Verification items for the finished model (mm, model axes). Give positions to 0.01 mm unless a question says otherwise; leave off trailing zeros. Write each loop counter-clockwise with the first axis right and the second up, starting at its lowest first coordinate (ties: lowest second). Pieces come first, ordered by that corner, then holes. Notation, with made-up numbers: (24, 82) - (77, 82) arc R22 cw to (77, 113) - close; hole circle Ø3 at (-22, 51). An arc over 180 degrees is marked (long way). Put each result on its own line as item: value.
from build123d import *

# Parameters (mm, degrees)
SKETCH_R        = 17.5
SKETCH_R_2      = 8.85
SKETCH_R_3      = 2.6
PAD_DEPTH       = 5.2
SKETCH001_R     = 17.5
SKETCH001_R_2   = 8.85
PAD001_DEPTH    = 0.2
CHAMFER_SIZE    = 0.25
CHAMFER001_SIZE = 0.25


with BuildPart() as part:
    # Sketch → Pad (new body)
    with BuildSketch(Plane.XY):
        Circle(SKETCH_R)
        Circle(SKETCH_R_2, mode=Mode.SUBTRACT)
        with Locations((12.5, 0)):
            Circle(SKETCH_R_3, mode=Mode.SUBTRACT)
        with Locations((-12.5, 0)):
            Circle(SKETCH_R_3, mode=Mode.SUBTRACT)
        with Locations((-6.25, 10.825318)):
            Circle(SKETCH_R_3, mode=Mode.SUBTRACT)
        with Locations((6.25, 10.825318)):
            Circle(SKETCH_R_3, mode=Mode.SUBTRACT)
        with Locations((-6.25, -10.825318)):
            Circle(SKETCH_R_3, mode=Mode.SUBTRACT)
        with Locations((6.25, -10.825318)):
            Circle(SKETCH_R_3, mode=Mode.SUBTRACT)
    extrude(amount=PAD_DEPTH)

    # Sketch001 → Pad001 (join)
    with BuildSketch(Plane.XY):
        Circle(SKETCH001_R)
        Circle(SKETCH001_R_2, mode=Mode.SUBTRACT)
    extrude(amount=PAD001_DEPTH)

    # Chamfer
    chamfer_edges = [part.edges().sort_by_distance(p)[0] for p in [
        (-17.5, 0, 5.2),
        (-8.85, 0, 5.2),
        (3.65, -10.825318, 5.2),
        (-8.85, 10.825318, 5.2),
        (-15.1, 0, 5.2),
        (9.9, 0, 5.2),
        (-8.85, -10.825318, 5.2),
        (3.65, 10.825318, 5.2),
    ]]
    chamfer(chamfer_edges, length=CHAMFER_SIZE)

    # Chamfer001
    chamfer001_edges = [part.edges().sort_by_distance(p)[0] for p in [
        (-17.5, 0, 0),
        (-8.85, 0, 0),
    ]]
    chamfer(chamfer001_edges, length=CHAMFER001_SIZE)


solid = part.part
Q1. Section check B-B, the plane y = 0. Record the cut outline in (x, z), plus the area to 3 significant figures.
Answers follow:
outline: (-17.5, 0.25) - (-17.25, 0) - (-9.1, 0) - (-8.85, 0.25) - (-8.85, 4.95) - (-9.1, 5.2) - (-9.65, 5.2) - (-9.9, 4.95) - (-9.9, 0.2) - (-15.1, 0.2) - (-15.1, 4.95) - (-15.35, 5.2) - (-17.25, 5.2) - (-17.5, 4.95) - close; (8.85, 0.25) - (9.1, 0) - (17.25, 0) - (17.5, 0.25) - (17.5, 4.95) - (17.25, 5.2) - (15.35, 5.2) - (15.1, 4.95) - (15.1, 0.2) - (9.9, 0.2) - (9.9, 4.95) - (9.65, 5.2) - (9.1, 5.2) - (8.85, 4.95) - close
area: 37.6 mm2
Q2. Section check C-C, the plane z = 3.65. Record the cut outline in (x, y).
Answers follow:
outline: circle Ø35 at (0, 0); hole circle Ø5.2 at (-12.5, 0); hole circle Ø5.2 at (-6.25, -10.83); hole circle Ø17.7 at (0, 0); hole circle Ø5.2 at (-6.25, 10.83); hole circle Ø5.2 at (6.25, -10.83); hole circle Ø5.2 at (6.25, 10.83); hole circle Ø5.2 at (12.5, 0)
Q3. Section check A-A, the plane x = 0. Record the cut outline in (y, z).
Answers follow:
outline: (-17.5, 0.25) - (-17.25, 0) - (-9.1, 0) - (-8.85, 0.25) - (-8.85, 4.95) - (-9.1, 5.2) - (-17.25, 5.2) - (-17.5, 4.95) - close; (8.85, 0.25) - (9.1, 0) - (17.25, 0) - (17.5, 0.25) - (17.5, 4.95) - (17.25, 5.2) - (9.1, 5.2) - (8.85, 4.95) - close
Q4. Scan lines: line 1 along Y through (x, z) = (0, 2.9); line 2 along X through (y, z) = (-12.5, 3.5); line 3 along Y through (x, z) = (6.25, 3.4). Record each from-to range of solid material in increasing order.
Answers follow:
line 1: y = -17.5 to -8.85, 8.85 to 17.5
line 2: x = -12.25 to -8.24, -4.26 to 4.26, 8.24 to 12.25
line 3: y = -16.35 to -13.43, -8.23 to -6.27, 6.27 to 8.23, 13.43 to 16.35
Q5. Go/stop test with flat-tipped pins: pin 1 Ø2.5 at (x, y) = (-13, 0) entering from +Z; pin 2 Ø1 at (x, z) = (8.5, 1.5) entering from -Y; pin 3 Ø5.5 at (x, y) = (12.5, 0) entering from +Z; pin 4 Ø2 at (x, y) = (-5.5, 5) entering from +Z. Record where each tip stops, or that it passes through.
Answers follow:
pin 1: stops at z = 0.2
pin 2: stops at y = -15.56
pin 3: stops at z = 5.1
pin 4: passes through
Q6. Release check for a two-part mould opening along Y. For faces 1 (the face through (5.9, 13.4, 2.5)), 2 (the face through (7, -7, 5.2)), 3 (the face through (-13.887, -10.648, 2.567)) record: released by +Y, released by -Y, zero draft, split by the parting line, or undercut.
Answers follow:
face 1: undercut
face 2: zero draft
face 3: split by the parting line
